Source: three-view drawing plus pictorial views. Frame: mm from the lowest corner of the part. A direction names the side the tool comes from. Give positions to 0.01 mm unless a question says otherwise; leave off trailing zeros. Write each loop counter-clockwise with the first axis right and the second up, starting at its lowest first coordinate (ties: lowest second). Pieces come first, ordered by that corner, then holes. Notation, with made-up numbers: (-36, 19.25) -> (-18, 19.25) arc R17 ccw to (-18, 23.25) -> close; hole circle Ø4 at (-18, 85). An arc over 180 degrees is marked (long way). Answer in a Markdown table with one row per item. Add a question column.
Item 1: Section query D-D on y = 11.25. Output: boundary loops of the cut face in (x, z), plus the area to 3 significant figures.
Item 2: Material intervals for probe 1 along Z at (x, y) = (31.75, 5.5); probe 2 along Z at (x, y) = (31.75, 12.2); probe 3 along Z at (x, y) = (5, 11.5), sorted ascending. Write a range as from..to.
Item 3: First-contact query: P1, Ø4, axis at x = 59.5, y = 6.5, coming from the +Z side; P2, Ø5, axis at x = 29.5, z = 28.5, coming from the -Y side; P3, Ø1, axis at x = 17.5, y = 2, coming from the +Z side (1 decimal). Flat tips, straight axial feed; report the tip coordinate or a pass-through.
Item 4: Section query A-A on y = 6.35. Output: boundary loops of the cut face in (x, z).
Item 5: Section query B-B on x = 57.15. Output: boundary loops of the cut face in (y, z).
Item 6: Section query C-C on z = 46. Output: boundary loops of the cut face in (x, y) (1 decimal), plus the area to 3 significant figures.
Item 7: Access query for the marked faces 1, 2 and 3. Directions: +Z, -Z, +X, -X, +Y, -Y. A direction counts if a zero-diameter tool reaches every point of the face in a straight line with its end or side. Return the directions, or none.
Item 8: Draft query along Z for the marked faces 4, 5 and 6. Return one class per face: +Z half, -Z half, draft (parallel to the pull), parting line (faces both ways), or undercut.
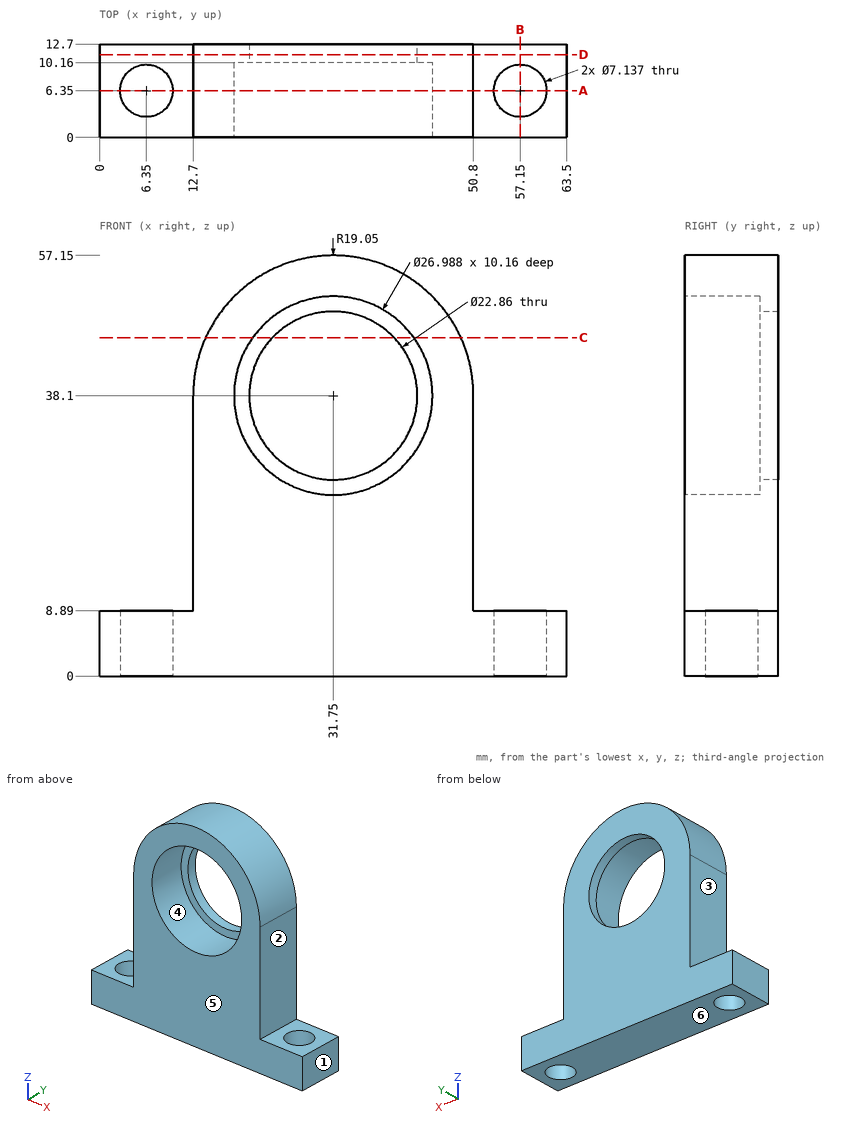
Findings below:
| question | item | result |
|---|---|---|
| 1 | outline | (0, 0) -> (63.5, 0) -> (63.5, 8.89) -> (50.8, 8.89) -> (50.8, 38.1) arc R19.05 ccw to (12.7, 38.1) -> (12.7, 8.89) -> (0, 8.89) -> close; hole circle Ø22.86 at (31.75, 38.1) |
| 1 | area | 1,840 mm^2 |
| 2 | probe 1 | z = 0..24.61, 51.59..57.15 |
| 2 | probe 2 | z = 0..26.67, 49.53..57.15 |
| 2 | probe 3 | z = 0..8.89 |
| 3 | P1 | stops at z = 8.89 |
| 3 | P2 | stops at y = 10.16 |
| 3 | P3 | stops at z = 51.3 |
| 4 | outline | (0, 0) -> (2.78, 0) -> (2.78, 8.89) -> (0, 8.89) -> close; (9.92, 0) -> (53.58, 0) -> (53.58, 8.89) -> (50.8, 8.89) -> (50.8, 38.1) arc R19.05 ccw to (12.7, 38.1) -> (12.7, 8.89) -> (9.92, 8.89) -> close; (60.72, 0) -> (63.5, 0) -> (63.5, 8.89) -> (60.72, 8.89) -> close; hole circle Ø26.99 at (31.75, 38.1) |
| 5 | outline | (0, 0) -> (2.78, 0) -> (2.78, 8.89) -> (0, 8.89) -> close; (9.92, 0) -> (12.7, 0) -> (12.7, 8.89) -> (9.92, 8.89) -> close |
| 6 | outline | (14.4, 0) -> (20.8, 0) -> (20.8, 10.2) -> (23.5, 10.2) -> (23.5, 12.7) -> (14.4, 12.7) -> close; (40, 10.2) -> (42.7, 10.2) -> (42.7, 0) -> (49.1, 0) -> (49.1, 12.7) -> (40, 12.7) -> close |
| 6 | area | 176 mm^2 |
| 7 | face 1 | +Z, -Z, +X, +Y, -Y |
| 7 | face 2 | +Z, +X, +Y, -Y |
| 7 | face 3 | +Z, -X, +Y, -Y |
| 8 | face 4 | undercut |
| 8 | face 5 | draft |
| 8 | face 6 | -Z half |
